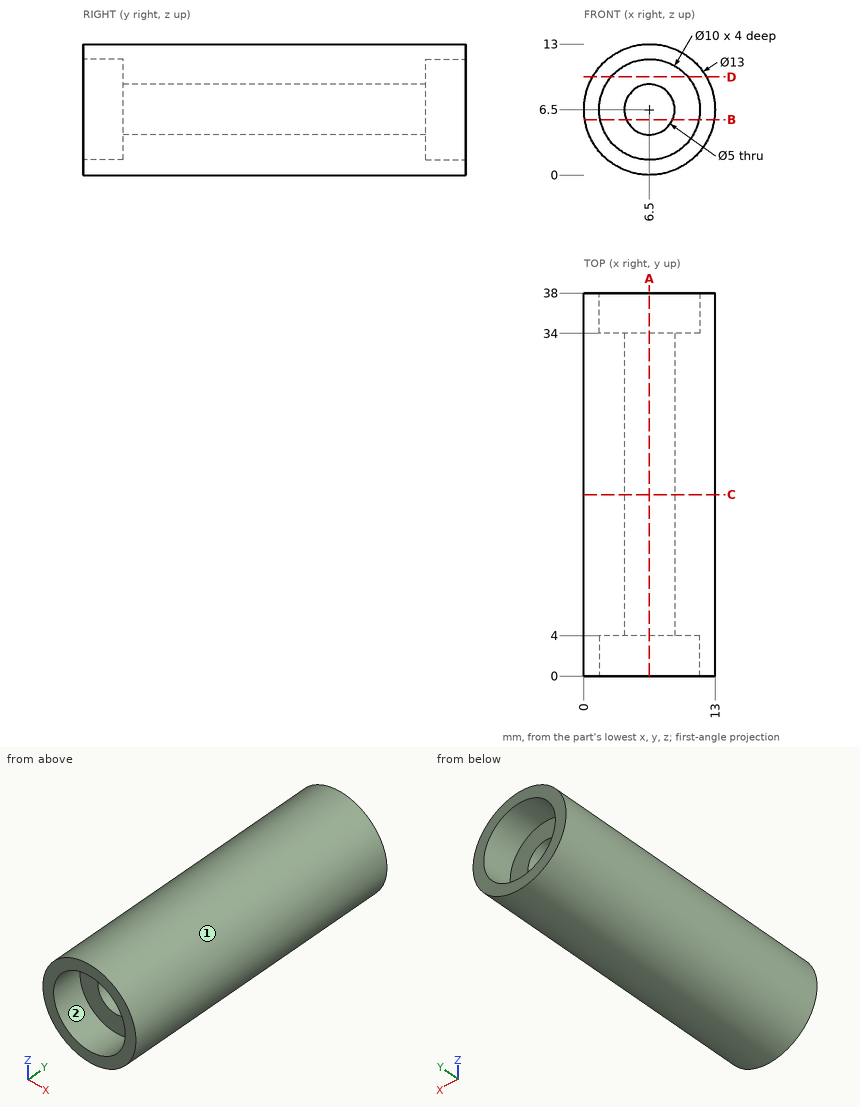
Source: three-view drawing plus pictorial views. Frame: mm from the lowest corner of the part. Round coordinates to 2 decimals unless told otherwise and drop trailing zeros. Write each loop counter-clockwise with the first axis right and the second up, starting at its lowest first coordinate (ties: lowest second). Pieces come first, ordered by that corner, then holes. Notation, with made-up numbers: M 31.5,-6 L 52.5,-6 A34 ccw 52.5,33 Z; hole C -21,8 d9. An arc over 180 degrees is marked long. One line per item, written item: value. Start each with the question number.
Item 1: Pin query (flat end, axial travel): pin 1 (4 mm diameter, centred on y = 24.5, z = 9, fed in from +X); pin 2 (2 mm diameter, centred on x = 8.5, z = 9, fed in from +Y); pin 3 (1.5 mm diameter, centred on x = 1.5, y = 8.5, fed in from +Z); pin 4 (4 mm diameter, centred on x = 6.5, z = 6.5, fed in from -Y). Return the tip coordinate at first contact, or that it passes through.
Item 2: Ray query, L1, parallel to Z at x = 6.5, y = 35.8; L2, parallel to Z at x = 6.5, y = 26.5. Return the intervals inside material, ascending. Write a range as from..to.
Item 3: Section query D-D (z = 9.75). Return the cut outline in (x, y), plus the area to 3 significant figures.
Item 4: Mould query, pull axis X, two halves, no side actions, for the marked faces 1 and 2. Classes: pulls with the +X half, pulls with the -X half, needs draft (parallel to the pull), parting line crosses it, or undercut.
Item 5: Section query A-A (x = 6.5). Return the cut outline in (y, z), plus the area to 3 significant figures.
Item 6: Section query B-B (z = 5.5). Return the cut outline in (x, y).
Item 7: Section query C-C (y = 18). Return the cut outline in (x, z), plus the area to 3 significant figures.
Result set:
1. pin 1: stops at x = 12.98
1. pin 2: stops at y = 34
1. pin 3: stops at z = 11.42
1. pin 4: passes through
2. L1: z = 0..1.5, 11.5..13
2. L2: z = 0..4, 9..13
3. outline: M 0.87,0 L 2.7,0 L 2.7,4 L 10.3,4 L 10.3,0 L 12.13,0 L 12.13,38 L 10.3,38 L 10.3,34 L 2.7,34 L 2.7,38 L 0.87,38 Z
3. area: 367 mm²
4. face 1: parting line crosses it
4. face 2: undercut
5. outline: M 0,0 L 38,0 L 38,1.5 L 34,1.5 L 34,4 L 4,4 L 4,1.5 L 0,1.5 Z; M 0,11.5 L 4,11.5 L 4,9 L 34,9 L 34,11.5 L 38,11.5 L 38,13 L 0,13 Z
5. area: 264 mm²
6. outline: M 0.08,0 L 1.6,0 L 1.6,4 L 4.21,4 L 4.21,34 L 1.6,34 L 1.6,38 L 0.08,38 Z; M 8.79,4 L 11.4,4 L 11.4,0 L 12.92,0 L 12.92,38 L 11.4,38 L 11.4,34 L 8.79,34 Z
7. outline: C 6.5,6.5 d13; hole C 6.5,6.5 d5
7. area: 113 mm²
